from build123d import *

# Parameters (mm, degrees)
EXTRUDE_1_DEPTH          = 25
SKETCH_2_W               = 7.514045852
SKETCH_2_H               = 2.645790793
CUT_EXTRUDE_1_DEPTH      = 109
CUT_EXTRUDE_1_DEPTH_BACK = 54
SKETCH_3_R               = 1.5
CUT_EXTRUDE_2_DEPTH      = 7
CUT_EXTRUDE_START        = -2
CUT_EXTRUDE_3_DEPTH      = 21
CUT_EXTRUDE_4_DEPTH      = 1.5


with BuildPart() as part:
    # 草图1 → 凸台-拉伸1 (new body)
    with BuildSketch(Plane.XY):
        with BuildLine():
            Line((30, -32), (-30, -32))
            Line((-30, -32), (-30, -29))
            Line((-30, -29), (-13.527749258, -29))
            ThreePointArc((-13.527749258, -29), (-23.208811843, -22.030684348), (-29.664793948, -12))
            Line((-29.664793948, -12), (-24.186773245, -12))
            ThreePointArc((-24.186773245, -12), (0, -27), (24.186773245, -12))
            Line((24.186773245, -12), (29.664793948, -12))
            ThreePointArc((29.664793948, -12), (23.208811843, -22.030684348), (13.527749258, -29))
            Line((13.527749258, -29), (30, -29))
            Line((30, -29), (30, -32))
        make_face()
    extrude(amount=EXTRUDE_1_DEPTH)

    # 草图2 → 切除-拉伸1 (cut, two sides)
    with BuildSketch(Plane(origin=(0, 0, 0), x_dir=(0, 0, -1), z_dir=(1, 0, 0))) as cut_extrude_1_sk:
        with Locations((-12.5, -16.322895397)):
            Rectangle(SKETCH_2_W, SKETCH_2_H)
    extrude(amount=CUT_EXTRUDE_1_DEPTH, mode=Mode.SUBTRACT)
    extrude(cut_extrude_1_sk.sketch, amount=-CUT_EXTRUDE_1_DEPTH_BACK, mode=Mode.SUBTRACT)

    # 草图3 → 切除-拉伸2 (cut)
    with BuildSketch(Plane.XZ.offset(32)):
        with Locations((-25, 20)):
            Circle(SKETCH_3_R)
        with Locations((25, 20)):
            Circle(SKETCH_3_R)
        with Locations((25, 5)):
            Circle(SKETCH_3_R)
        with Locations((-25, 5)):
            Circle(SKETCH_3_R)
    extrude(amount=-CUT_EXTRUDE_2_DEPTH, mode=Mode.SUBTRACT)

    # 草图4 → 切除-拉伸3 (cut)
    with BuildSketch(Plane.XY.offset(25).offset(CUT_EXTRUDE_START)):
        with BuildLine():
            Line((24.186773245, -12), (25.298221281, -12))
            ThreePointArc((25.298221281, -12), (0, -28), (-25.298221281, -12))
            Line((-25.298221281, -12), (-24.186773245, -12))
            ThreePointArc((-24.186773245, -12), (0, -27), (24.186773245, -12))
        make_face()
    extrude(amount=-CUT_EXTRUDE_3_DEPTH, mode=Mode.SUBTRACT)

    # 草图5 → 切除-拉伸4 (cut)
    with BuildSketch(Plane(origin=(0, -29, 0), x_dir=(1, 0, 0), z_dir=(0, 1, 0))):
        Polygon((-25, -23.290896534), (-22.15, -21.645448267), (-22.15, -18.354551733), (-25, -16.709103466), (-27.85, -18.354551733), (-27.85, -21.645448267), align=None)
        Polygon((27.85, -21.645448267), (25, -23.290896534), (22.15, -21.645448267), (22.15, -18.354551733), (25, -16.709103466), (27.85, -18.354551733), align=None)
        Polygon((25, -1.709103466), (22.15, -3.354551733), (22.15, -6.645448267), (25, -8.290896534), (27.85, -6.645448267), (27.85, -3.354551733), align=None)
        Polygon((-27.85, -3.354551733), (-25, -1.709103466), (-22.15, -3.354551733), (-22.15, -6.645448267), (-25, -8.290896534), (-27.85, -6.645448267), align=None)
    extrude(amount=-CUT_EXTRUDE_4_DEPTH, mode=Mode.SUBTRACT)


solid = part.part
Geometry check sheet. Reference: the model listing, model coordinates, mm. A direction names the side the tool comes from. Round coordinates to 2 decimals unless told otherwise and drop trailing zeros. Order: outer loops, then holes, each group sorted by start corner. A loop starts at its lowest first (then second) coordinate and runs counter-clockwise, first axis right, second up. Notation, with made-up numbers: (84, -35) -> (143, -35) arc R33 ccw to (143, -2) -> close; hole circle Ø6 at (44.5, -33). An arc over 180 degrees is marked (long way). Use one line per item in the form item = value.
1. Set-up check for faces 1 (the face through (-24, -17.646, 13)), 2 (the face through (26.44, -29.74, 2.54)), 3 (the face through (-26.11, -31.26, 21.01)): record each of +Z, -Z, +X, -X, +Y, -Y from which the full face is reachable in a straight line by a thin tool's end or side.
Working result:
face_1 = +X, -X
face_2 = none
face_3 = -Y
2. Go/stop test with flat-tipped pins: pin 1 (5 mm diameter, centred on x = 19, z = 17, fed in from +Y); pin 2 (1.5 mm diameter, centred on x = -24, z = 11.5, fed in from +Y). Record where each tip stops, or that it passes through.
Working result:
pin_1 = -17.94
pin_2 = -13.09
3. Cross-section at B-B, the plane y = -29.75. Enter the section's corners in (x, z), plus the area to 3 significant figures.
Working result:
outline = (-30, 0) -> (30, 0) -> (30, 25) -> (-30, 25) -> close; hole (-27.85, 3.35) -> (-25, 1.71) -> (-22.15, 3.35) -> (-22.15, 6.65) -> (-25, 8.29) -> (-27.85, 6.65) -> close; hole (-27.85, 18.35) -> (-25, 16.71) -> (-22.15, 18.35) -> (-22.15, 21.65) -> (-25, 23.29) -> (-27.85, 21.65) -> close; hole (22.15, 3.35) -> (25, 1.71) -> (27.85, 3.35) -> (27.85, 6.65) -> (25, 8.29) -> (22.15, 6.65) -> close; hole (22.15, 18.35) -> (25, 16.71) -> (27.85, 18.35) -> (27.85, 21.65) -> (25, 23.29) -> (22.15, 21.65) -> close
area = 1,390 mm^2
4. Scan lines: line 1 along Z through (x, y) = (25, -31.1); line 2 along X through (y, z) = (-18.25, 2.5); line 3 along Y through (x, z) = (15.5, 11.5). Record each from-to range of solid material in increasing order. Write a range as from..to.
Working result:
line_1 = 0..3.5, 6.5..18.5, 21.5..25
line_2 = -26.29..-21.24, 21.24..26.29
line_3 = -32..-29, -28..-23.32
5. Cross-section at C-C, the plane x = 19.5. Enter the section's corners in (y, z).
Working result:
outline = (-32, 0) -> (-29, 0) -> (-29, 25) -> (-32, 25) -> close; (-25.37, 0) -> (-18.67, 0) -> (-18.67, 2) -> (-20.09, 2) -> (-20.09, 23) -> (-18.67, 23) -> (-18.67, 25) -> (-25.37, 25) -> close
6. Cross-section at A-A, the plane z = 15.25. Enter the section's corners in (x, y).
Working result:
outline = (-30, -32) -> (30, -32) -> (30, -29) -> (13.53, -29) arc R32 ccw to (26.7, -17.65) -> (21.74, -17.65) arc R28 cw to (-21.74, -17.65) -> (-26.7, -17.65) arc R32 ccw to (-13.53, -29) -> (-30, -29) -> close; (-29.66, -12) arc R32 ccw to (-28.27, -15) -> (-23.64, -15) arc R28 cw to (-25.3, -12) -> close; (23.64, -15) -> (28.27, -15) arc R32 ccw to (29.66, -12) -> (25.3, -12) arc R28 cw to start
7. Mould release check, pull along Z, two halves, no side actions. Record for faces 4 (the face through (0, -29, 0)), 5 (the face through (25, -30.5, 18)), 6 (the face through (-22, -29, 12)): pulls with the +Z half, pulls with the -Z half, needs draft (parallel to the pull), parting line crosses it, or undercut.
Working result:
face_4 = pulls with the -Z half
face_5 = undercut
face_6 = needs draft
8. Cross-section at D-D, the plane y = -16.75. Enter the section's corners in (x, z).
Working result:
outline = (-27.27, 0) -> (-21.18, 0) -> (-21.18, 2) -> (-22.44, 2) -> (-22.44, 8.74) -> (-27.27, 8.74) -> close; (-27.27, 16.26) -> (-22.44, 16.26) -> (-22.44, 23) -> (-21.18, 23) -> (-21.18, 25) -> (-27.27, 25) -> close; (21.18, 0) -> (27.27, 0) -> (27.27, 8.74) -> (22.44, 8.74) -> (22.44, 2) -> (21.18, 2) -> close; (21.18, 23) -> (22.44, 23) -> (22.44, 16.26) -> (27.27, 16.26) -> (27.27, 25) -> (21.18, 25) -> close
